```python
from build123d import *

# Parameters (mm, degrees)
BOSS_EXTRUDE1_DEPTH      = 57.15
BOSS_EXTRUDE1_DEPTH_BACK = 44.45
SKETCH3_R                = 3.556
CUT_EXTRUDE1_DEPTH       = 13.7
SKETCH4_R                = 3.556
CUT_EXTRUDE2_DEPTH       = 13.7


with BuildPart() as part:
    # Sketch1 → Boss-Extrude1 (new body, two sides)
    with BuildSketch(Plane(origin=(0, 0, 0), x_dir=(0, 0, -1), z_dir=(1, 0, 0))) as boss_extrude1_sk:
        Polygon((0, 0), (0, 12.7), (-12.7, 12.7), (-12.7, 11.1125), (-1.5875, 11.1125), (-1.5875, 0), align=None)
    extrude(amount=BOSS_EXTRUDE1_DEPTH)
    extrude(boss_extrude1_sk.sketch, amount=-BOSS_EXTRUDE1_DEPTH_BACK)

    # Sketch3 → Cut-Extrude1 (cut, through all)
    with BuildSketch(Plane(origin=(0, 0, 0), x_dir=(-1, 0, 0), z_dir=(0, 0, -1))):
        with Locations((25.4, 5.08)):
            Circle(SKETCH3_R)
        with Locations((-50.8, 5.08)):
            Circle(SKETCH3_R)
    extrude(amount=-CUT_EXTRUDE1_DEPTH, mode=Mode.SUBTRACT)

    # Sketch4 → Cut-Extrude2 (cut, through all)
    with BuildSketch(Plane(origin=(0, 12.7, 0), x_dir=(1, 0, 0), z_dir=(0, 1, 0))):
        with Locations((-38.1, -7.62)):
            Circle(SKETCH4_R)
        with Locations((38.1, -7.62)):
            Circle(SKETCH4_R)
    extrude(amount=-CUT_EXTRUDE2_DEPTH, mode=Mode.SUBTRACT)


solid = part.part
```
Part model, mm, in its own coordinate system. A direction names the side the tool comes from. Round coordinates to 2 decimals unless told otherwise and drop trailing zeros. Write each loop counter-clockwise with the first axis right and the second up, starting at its lowest first coordinate (ties: lowest second). Pieces come first, ordered by that corner, then holes. Notation, with made-up numbers: M -18.75,7 L 4.25,7 A26 ccw 4.25,44 Z; hole C 42,36 d10. An arc over 180 degrees is marked long. One line per question, with ' | ' between items.
(1) Saw through at B-B on y = 5.08. Write the cut outline in (x, z).
Answer key:
outline: M -44.45,0 L -28.96,0 L -28.96,1.59 L -44.45,1.59 Z; M -21.84,0 L 47.24,0 L 47.24,1.59 L -21.84,1.59 Z; M 54.36,0 L 57.15,0 L 57.15,1.59 L 54.36,1.59 Z
(2) Saw through at A-A on z = 7.62. Write the cut outline in (x, y).
Answer key:
outline: M -44.45,11.11 L -41.66,11.11 L -41.66,12.7 L -44.45,12.7 Z; M -34.54,11.11 L 34.54,11.11 L 34.54,12.7 L -34.54,12.7 Z; M 41.66,11.11 L 57.15,11.11 L 57.15,12.7 L 41.66,12.7 Z
(3) Probe line 1 along X through (y, z) = (12.1, 7.62); line 2 along Y through (x, z) = (-25.4, 0.4); line 3 along Z through (x, y) = (-34, 7.5). List the from-to ranges inside material, lowest first.
Answer key:
line 1: x = -44.45 to -41.66, -34.54 to 34.54, 41.66 to 57.15 | line 2: y = 0 to 1.52, 8.64 to 12.7 | line 3: z = 0 to 1.59
(4) Saw through at D-D on x = -36. Write the cut outline in (y, z).
Answer key:
outline: M 0,0 L 12.7,0 L 12.7,4.75 L 11.11,4.75 L 11.11,1.59 L 0,1.59 Z; M 11.11,10.49 L 12.7,10.49 L 12.7,12.7 L 11.11,12.7 Z
(5) Saw through at C-C on x = -25.4. Write the cut outline in (y, z), then the cut area to 3 significant figures.
Answer key:
outline: M 0,0 L 1.52,0 L 1.52,1.59 L 0,1.59 Z; M 8.64,0 L 12.7,0 L 12.7,12.7 L 11.11,12.7 L 11.11,1.59 L 8.64,1.59 Z | area: 26.5 mm^2
(6) Pin check, flat tips, straight feed: pin 1 (3.5 mm diameter, centred on x = 27, z = 5, fed in from -Y); pin 2 (4.5 mm diameter, centred on x = -38.1, z = 7.62, fed in from +Y). Stop position of each tip, or through.
Answer key:
pin 1: stops at y = 11.11 | pin 2: passes through
(7) 3-axis set-ups, long thin cutter, end or side, ignore diameter. For faces 1 (the face through (7, 6, 1.588)), 2 (the face through (7, 12.7, 6)): which of +Z, -Z, +X, -X, +Y, -Y reach the whole face in a straight line?
Answer key:
face 1: +Z, +X, -X, -Y | face 2: +Z, -Z, +X, -X, +Y
(8) Two-plate mould, pull along X, no slides. Class faces 3 (the face through (-44.45, 12, 4)), 4 (the face through (-41.653, 11.917, 7.464)), 5 (the face through (7, 12, 12.7)): released by +X, released by -X, zero draft, split by the parting line, or undercut.
Answer key:
face 3: released by -X | face 4: undercut | face 5: zero draft
